```python
from build123d import *

# Parameters (mm, degrees)
SKETCH1_W           = 25.4
SKETCH1_H           = 101.6
BOSS_EXTRUDE1_DEPTH = 1.5875
FILLET2_R           = 6.35
CUT_EXTRUDE1_REACH  = 54.388
SKETCH2_R           = 4.165


with BuildPart() as part:
    # Sketch1 → Boss-Extrude1 (new body)
    with BuildSketch(Plane(origin=(0, 0, 0), x_dir=(1, 0, 0), z_dir=(0, 1, 0))):
        Rectangle(SKETCH1_W, SKETCH1_H)
    extrude(amount=BOSS_EXTRUDE1_DEPTH)

    # Fillet2
    fillet2_edges = [part.edges().sort_by_distance(p)[0] for p in [
        (12.7, 0.79375, 50.8),
        (12.7, 0.79375, -50.8),
    ]]
    fillet(fillet2_edges, radius=FILLET2_R)

    # Sketch2 → Cut-Extrude1 (cut, up to next)
    with BuildSketch(Plane(origin=(0, 1.5875, 0), x_dir=(1, 0, 0), z_dir=(0, 1, 0)), mode=Mode.PRIVATE) as cut_extrude1_sk1:
        with Locations(Location((2.7, 38.1, 0), (0, 0, 270))):
            Circle(SKETCH2_R)
    cut_extrude1_tool1 = extrude(cut_extrude1_sk1.sketch, amount=-CUT_EXTRUDE1_REACH, mode=Mode.PRIVATE) & part.part
    # Sketch2 → Cut-Extrude1 (cut, up to next)
    with BuildSketch(Plane(origin=(0, 1.5875, 0), x_dir=(1, 0, 0), z_dir=(0, 1, 0)), mode=Mode.PRIVATE) as cut_extrude1_sk2:
        with Locations(Location((2.7, -38.1, 0), (0, 0, 270))):
            Circle(SKETCH2_R)
    cut_extrude1_tool2 = extrude(cut_extrude1_sk2.sketch, amount=-CUT_EXTRUDE1_REACH, mode=Mode.PRIVATE) & part.part
    add(cut_extrude1_tool1.solids().sort_by_distance((2.7, 1.5875, -38.1))[0], mode=Mode.SUBTRACT)
    add(cut_extrude1_tool2.solids().sort_by_distance((2.7, 1.5875, 38.1))[0], mode=Mode.SUBTRACT)


solid = part.part
```
Can you work these out from the model? Positions are in its coordinate system, mm. Round coordinates to 2 decimals unless told otherwise and drop trailing zeros. Loops run counter-clockwise (first coordinate to the right, second up) from the corner with the lowest first, then second, coordinate; pieces in that order, holes last. Notation, with made-up numbers: (78.5, 75.5) -> (104.5, 75.5) arc R25 ccw to (104.5, 90.5) -> close; hole circle Ø5 at (75.25, 10.5). An arc over 180 degrees is marked (long way). One line per item, written item: value. Start each with the question number.
1. If we mould it in two halves opening along X, with no side actions, what happens to faces 1 (the flat face through (-12.7, 1, 1)), 2 (the cylindrical face through (2.88, 0.8, -42.26)), 3 (the cylindrical face through (1.105, 0.805, 41.947)), 4 (the flat face through (0, 1.588, -1))? For each: pulls with the +X half, pulls with the -X half, needs draft (parallel to the pull), parting line crosses it, or undercut.
2. For pin 1 (6.5 mm diameter, centred on x = 2.7, z = 38.1, fed in from +Y), with a flat end and sliding along its axis, tell me the tip position at first contact or that it passes through.
3. If we section it at A-A, the plane z = 38.1: Write out the boundary of the cut face in (x, y) (1 decimal), then the cut area to 3 significant figures.
4. If I drill on probe 1 along Z at (x, y) = (2.5, 0.15); probe 2 along Z at (x, y) = (2, 0.7); probe 3 along X at (y, z) = (0.45, 38.1) (3 decimals), over which ranges is the centre line in solid material (lowest first)?
5. If we section it at B-B, the plane x = 0.25: Write out the boundary of the cut face in (y, z).
6. If we section it at C-C, the plane y = 1.3: Write out the boundary of the cut face in (x, z) (3 decimals).
Calculated:
1. face 1: pulls with the -X half
1. face 2: undercut
1. face 3: undercut
1. face 4: needs draft
2. pin 1: passes through
3. outline: (-12.7, 0) -> (-1.5, 0) -> (-1.5, 1.6) -> (-12.7, 1.6) -> close; (6.9, 0) -> (12.7, 0) -> (12.7, 1.6) -> (6.9, 1.6) -> close
3. area: 27.1 mm²
4. probe 1: z = -50.8 to -42.26, -33.94 to 33.94, 42.26 to 50.8
4. probe 2: z = -50.8 to -42.21, -33.99 to 33.99, 42.21 to 50.8
4. probe 3: x = -12.7 to -1.465, 6.865 to 12.7
5. outline: (0, -50.8) -> (1.59, -50.8) -> (1.59, -41.47) -> (0, -41.47) -> close; (0, -34.73) -> (1.59, -34.73) -> (1.59, 34.73) -> (0, 34.73) -> close; (0, 41.47) -> (1.59, 41.47) -> (1.59, 50.8) -> (0, 50.8) -> close
6. outline: (-12.7, -50.8) -> (6.35, -50.8) arc R6.35 ccw to (12.7, -44.45) -> (12.7, 44.45) arc R6.35 ccw to (6.35, 50.8) -> (-12.7, 50.8) -> close; hole circle Ø8.33 at (2.7, -38.1); hole circle Ø8.33 at (2.7, 38.1)
